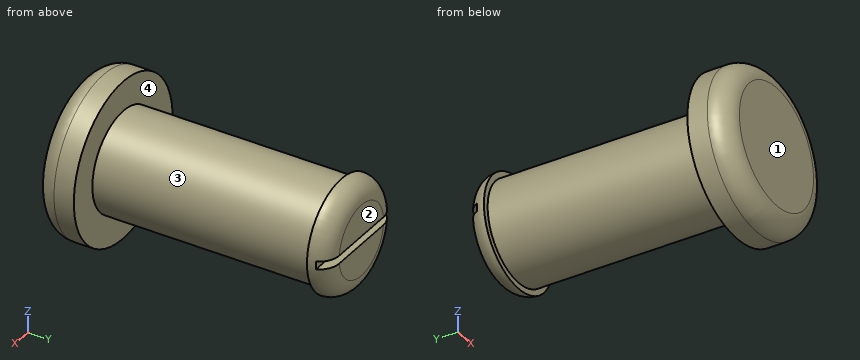
from build123d import *

# Parameters (mm, degrees)
F2_R     = 0.5
F3_R     = 0.49999
F4_W     = 3
F4_H     = 0.1
F5_DEPTH = 0.3


# Not quite as in the source:
# - a fillet or chamfer is up to 0.001 mm smaller than in the source, because OpenCascade refuses the exact size


with BuildPart() as f1:
    # F0 (on Right) → F1 (revolve)
    with BuildSketch(Plane.YZ):
        Polygon((-3.5, 0), (-2.5, 0), (3, 0), (3.5, 0), (3.5, 1.4), (3, 1.4), (3, 1.25), (-2.5, 1.25), (-2.5, 2), (-3.5, 2), align=None)
    revolve(axis=Axis((0, 0.25, 0), (0, -1, 0)))

    # F2
    f2_edges = [f1.edges().sort_by_distance(p)[0] for p in [
        (0, -3.5, -2),
    ]]
    fillet(f2_edges, radius=F2_R)

    # F3 (radius 0.5 in the source; OpenCascade refuses exactly that, so slightly less here)
    f3_edges = [f1.edges().sort_by_distance(p)[0] for p in [
        (0, 3.5, -1.4),
    ]]
    fillet(f3_edges, radius=F3_R)

    # F4 (on face) → F5 (cut)
    with BuildSketch(Plane(origin=(0, 3.5, 0), x_dir=(-1, 0, 0), z_dir=(0, 1, 0))):
        with Locations((0, 0.05)):
            Rectangle(F4_W, F4_H)
        with Locations((0, -0.05)):
            Rectangle(F4_W, F4_H)
    extrude(amount=-F5_DEPTH, mode=Mode.SUBTRACT)


solid = f1.part
Build history of the part. All positions in model axes, mm. Face numbers are marked on the shaded views. Coordinates: 2 decimals unless noted, no trailing zeros. Order: outer loops, then holes, each group sorted by start corner. A loop starts at its lowest first (then second) coordinate and runs counter-clockwise, first axis right, second up. Notation, with made-up numbers: (30, -15.75) -> (71, -15.75) arc R15 ccw to (71, 4.25) -> close; hole circle Ø3 at (-24.75, -27.5). An arc over 180 degrees is marked (long way). One line per item, written item: value.
(1) Drop flat-ended pins along their axis: pin 1 Ø2 at (x, y) = (-1.5, 1.5) entering from +Z; pin 2 Ø2 at (y, z) = (-1, 1.5) entering from -X. Give the stop position or say it passes through.
Checked values:
pin 1: z = 1.15
pin 2: x = -1.15
(2) Probe line 1 (Y direction, x = -1.3, z = 0.2); line 2 (Z direction, x = 0.5, y = 3.25); line 3 (Y direction, x = -1.5, z = -0.3). List the from-to ranges inside material, lowest first. Write a range as [from, to].
Checked values:
line 1: [-3.5, -2.5], [3, 3.28]
line 2: [-1.24, -0.1], [0.1, 1.24]
line 3: [-3.5, -2.5]
(3) Slice it at C-C, the plane y = 0. List the corners of the cut face in (x, z), plus the area to 3 significant figures.
Checked values:
outline: circle Ø2.5 at (0, 0)
area: 4.91 mm2
(4) Mould opens along Y. For the marked faces 1, 2, 3 and 4 say: pulls with the +Y half, pulls with the -Y half, needs draft (parallel to the pull), parting line crosses it, or undercut.
Checked values:
face 1: pulls with the -Y half
face 2: pulls with the +Y half
face 3: undercut
face 4: undercut
